Autodesk Inventor part; units mm, degrees
ref_plane "YZ Plane" through (0, 0, 0) normal (1, 0, 0) x (0, 1, 0)
ref_plane "XZ Plane" through (0, 0, 0) normal (0, 1, 0) x (-1, 0, 0)
ref_plane "XY Plane" through (0, 0, 0) normal (0, 0, 1) x (1, 0, 0)
sketch "Sketch1" plane through (0, 0, 0) normal (0, 1, 0) x (-1, 0, 0)
  line L0 (-4.9492, -3.4256) -> (-7.9492, -3.4256)
  line L1 (-7.9492, -3.4256) -> (-7.9492, -13.4256)
  line L2 (-7.9492, -13.4256) -> (-4.9492, -13.4256)
  line L3 (-4.9492, -3.4256) -> (-4.9492, -0.4256)
  line L4 (-4.9492, -13.4256) -> (-4.9492, -16.4256)
  line L5 (-4.9492, -16.4256) -> (-2.8973, -16.4256)
  line L6 (-4.9492, -0.4256) -> (-2.8973, -0.4256)
  line L7 (91.2508, 106.8744) -> (94.2508, 106.8744)
  line L8 (94.2508, 106.8744) -> (94.2508, 96.8744)
  line L9 (94.2508, 96.8744) -> (91.2508, 96.8744)
  line L10 (91.2508, 106.8744) -> (91.2508, 109.8744)
  line L11 (91.2508, 96.8744) -> (91.2508, 93.8744)
  line L12 (91.2508, 93.8744) -> (89.1989, 93.8744)
  line L13 (91.2508, 109.8744) -> (89.1989, 109.8744)
  arc A0 (89.1989, 109.8744) -> (87.6506, 109.1404) centre (89.1989, 107.8744) ccw
  line L14 (-1.349, 0.3083) -> (87.6506, 109.1404)
  arc A1 (-2.8973, -0.4256) -> (-1.349, 0.3083) centre (-2.8973, 1.5744) ccw
  line L15 (-1.349, -15.6917) -> (87.6506, 93.1404)
  arc A2 (89.1989, 93.8744) -> (87.6506, 93.1404) centre (89.1989, 91.8744) ccw
  arc A3 (-2.8973, -16.4256) -> (-1.349, -15.6917) centre (-2.8973, -14.4256) ccw
  point P0 (0, 0)
extrude "Extrusion1" add sketch "Sketch1" along normal blind 3
properties part number "angularBrace" material "Polycarbonate, Clear"
The model under review builds one solid part; all positions refer to its coordinate system, in mm. A direction names the side the tool comes from. Round coordinates to 2 decimals unless told otherwise and drop trailing zeros. Order: outer loops, then holes, each group sorted by start corner. A loop starts at its lowest first (then second) coordinate and runs counter-clockwise, first axis right, second up. Notation, with made-up numbers: (81.25, 23.5) -> (132.25, 23.5) arc R27 cw to (132.25, 55.5) -> close; hole circle Ø8 at (80.25, -24.5). An arc over 180 degrees is marked (long way). One line per item, written item: value. Start each with the question number.
Q1. Take a section at C-C (z = 46). Write out the cut boundary in (x, y).
Q2. Wall thickness on line 1 (Z direction, x = -23, y = 2.45); line 2 (X direction, y = 0.1, z = 84.5); line 3 (X direction, y = 2.05, z = -3): over which ranges is each line inside the solid? List them lowest first.
Q3. Clearance check with flat-ended pins moving along their axes: pin 1 Ø0.6 at (x, y) = (4, 1.5) entering from +Z; pin 2 Ø1 at (y, z) = (1.5, 68) entering from -X; pin 3 Ø1.5 at (x, y) = (6.5, 1) entering from -Z. State where each tip first meets the part, or that it passes through.
Q4. Take a section at A-A (y = 1.8). Write out the cut boundary in (x, z).
Q5. Take a section at B-B (x = -31.5). Write out the cut boundary in (y, z), and give its area (3 significant figures).
Q6. Machinability: for faces 1 (the face through (4.949, 1, -2)), 2 (the face through (-93, 1, 106.874)), 3 (the face through (-93, 1, 96.874)), which of the approach directions +Z, -Z, +X, -X, +Y, -Y give a long, thin tool a straight path to every point of the face, cutting with its end or side? Answer none if there is none.
Reported:
1. outline: (-49.1, 0) -> (-36.02, 0) -> (-36.02, 3) -> (-49.1, 3) -> close
2. line 1: z = 14.08 to 30.08
2. line 2: x = -80.58 to -67.5
2. line 3: x = -9.03 to 4.95
3. pin 1: stops at z = -0.43
3. pin 2: stops at x = -67.5
3. pin 3: stops at z = -13.43
4. outline: (-94.25, 96.87) -> (-91.25, 96.87) -> (-91.25, 93.87) -> (-89.2, 93.87) arc R2 cw to (-87.65, 93.14) -> (1.35, -15.69) arc R2 ccw to (2.9, -16.43) -> (4.95, -16.43) -> (4.95, -13.43) -> (7.95, -13.43) -> (7.95, -3.43) -> (4.95, -3.43) -> (4.95, -0.43) -> (2.9, -0.43) arc R2 cw to (1.35, 0.31) -> (-87.65, 109.14) arc R2 ccw to (-89.2, 109.87) -> (-91.25, 109.87) -> (-91.25, 106.87) -> (-94.25, 106.87) -> close
5. outline: (0, 24.48) -> (3, 24.48) -> (3, 40.48) -> (0, 40.48) -> close
5. area: 48.0 mm2
6. face 1: +Z, +X, +Y, -Y
6. face 2: +Z, -X, +Y, -Y
6. face 3: -Z, -X, +Y, -Y
